Read the model definition and answer for the solid it produces. Units are mm, in the model's axes. Face numbers are marked on the shaded views. A direction names the side the tool comes from. Coordinates: 2 decimals unless noted, no trailing zeros. Write each loop counter-clockwise with the first axis right and the second up, starting at its lowest first coordinate (ties: lowest second). Pieces come first, ordered by that corner, then holes.
Item 1: Section C-C (x = -0.5) is taken. Give the vertices of the cut face in (y, z).
Item 2: Section D-D (x = 4.25) is taken. Give the vertices of the cut face in (y, z).
Item 3: Determine the mould class of the marked faces 1, 2 and 3 for opening direction Z: released by +Z, released by -Z, zero draft, split by the parting line, or undercut.
Item 4: Section B-B (x = 3.25) is taken. Give the vertices of the cut face in (y, z).
Item 5: Straight lines are drawn through the part: probe 1 along Z at (x, y) = (2.15, 0); probe 2 along Y at (x, z) = (5.5, -0.5); probe 3 along Y at (x, z) = (0.75, -1.5). For each, find the intervals that lie inside material, in ascending order.
Item 6: A tool of negligible diameter and unlimited length cuts with its end or side. For the marked faces 4, 5 and 6, from which of +Z, -Z, +X, -X, +Y, -Y can it reach the whole face along a straight path? Write none if from no direction.
Item 7: Each of these flat-tipped pins is pushed along its axis until it touches: P1, Ø3, axis at x = 3, z = -2.5, coming from the +Y side; P2, Ø1, axis at x = 4.5, z = -2.5, coming from the -Y side; P3, Ø1, axis at x = 4, y = 0.5, coming from the +Z side; P4, Ø2, axis at y = 0, z = 0, coming from the +X side. Where does it stop, or does it pass through?
from build123d import *

# Parameters (mm, degrees)
F2_R      = 3.1496
F3_DEPTH  = 5.969
F4_R      = 2.159
F5_DEPTH  = 8.9662
F0_R      = 1.7145
F6_DEPTH  = 3.7592
F8_DEPTH  = 12.7
F1_R      = 3.4925
F9_DEPTH  = 1.905
F10_DEPTH = 2.54
F11_SIZE  = 1.524


with BuildPart() as f3:
    # F2 (on Right) → F3 (new body)
    with BuildSketch(Plane.YZ):
        Circle(F2_R)
    extrude(amount=F3_DEPTH)

    # F4 (on Right) → F5 (cut)
    with BuildSketch(Plane.YZ):
        Circle(F4_R)
    extrude(amount=F5_DEPTH, mode=Mode.SUBTRACT)

    # F0 (on Right) → F6 (cut)
    with BuildSketch(Plane.YZ):
        Circle(F0_R)
    extrude(amount=-F6_DEPTH, mode=Mode.SUBTRACT)

    # F7 (on Top) → F8 (cut, symmetric)
    with BuildSketch(Plane.XY):
        Polygon((6.593515, 0.784034), (2.462917, 0.784034), (2.47918, 0), (6.593515, -1.02107), align=None)
    extrude(amount=F8_DEPTH, both=True, mode=Mode.SUBTRACT)

    # F1 (on Right) → F9 (join)
    with BuildSketch(Plane.YZ):
        Circle(F1_R)
    extrude(amount=-F9_DEPTH)

    # F0 (on Right) → F10 (cut)
    with BuildSketch(Plane.YZ):
        Circle(F0_R)
    extrude(amount=-F10_DEPTH, mode=Mode.SUBTRACT)

    # F11
    f11_edges = [f3.edges().sort_by_distance(p)[0] for p in [
        (-1.905, -3.4925, 0),
    ]]
    chamfer(f11_edges, length=F11_SIZE)


solid = f3.part
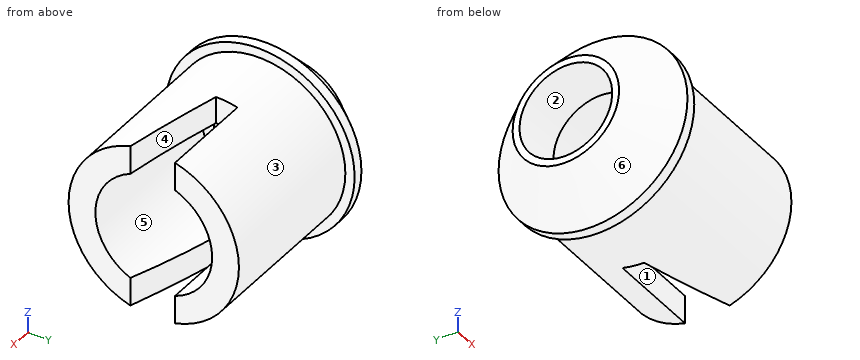
Established:
1. outline: circle Ø6.75 at (0, 0); hole circle Ø3.43 at (0, 0)
2. outline: (-0.44, -3.12) - (-0.44, -2.11) arc R2.16 cw to (-0.44, 2.11) - (-0.44, 3.12) arc R3.15 ccw to start; (0.78, -3.05) arc R3.15 ccw to (0.78, 3.05) - (0.78, 2.01) arc R2.16 cw to (0.78, -2.01) - close
3. face 1: zero draft
3. face 2: undercut
3. face 3: split by the parting line
4. outline: (-0.19, -3.14) - (-0.19, -2.15) arc R2.16 cw to (-0.19, 2.15) - (-0.19, 3.14) arc R3.15 ccw to start; (0.78, -3.05) arc R3.15 ccw to (0.78, 3.05) - (0.78, 2.01) arc R2.16 cw to (0.78, -2.01) - close
5. probe 1: z = -3.15 to -2.16, 2.16 to 3.15
5. probe 2: y = -3.11 to -2.1, 2.1 to 3.11
5. probe 3: y = -2.77 to -1.55, 1.55 to 2.77
6. face 4: +Z, -Z, +X
6. face 5: +X
6. face 6: -X
7. P1: stops at y = 2.99
7. P2: stops at y = -2.43
7. P3: stops at z = 3.05
7. P4: passes through
